The model under review builds one solid part; all positions refer to its coordinate system, in mm. Face numbers are marked on the shaded views. A direction names the side the tool comes from. Round coordinates to 2 decimals unless told otherwise and drop trailing zeros. Write each loop counter-clockwise with the first axis right and the second up, starting at its lowest first coordinate (ties: lowest second). Pieces come first, ordered by that corner, then holes. Notation, with made-up numbers: M 79.5,73.5 L 111.5,73.5 A27 cw 111.5,94.5 Z; hole C 20,-12.5 d8. An arc over 180 degrees is marked long. Write item = value, one per line. Start each with the question number.
Item 1: Take a section at B-B, the plane x = 0. Give the boundary of the cut face in (y, z), plus the area to 3 significant figures.
Item 2: Take a section at A-A, the plane y = 0. Give the boundary of the cut face in (x, z).
Item 3: For pin 1 Ø1.5 at (y, z) = (1, 18.5) entering from +X; pin 2 Ø1.5 at (x, y) = (0.5, 6.5) entering from +Z; pin 3 Ø9.5 at (x, y) = (0, 0) entering from -Z; pin 4 Ø1 at (x, z) = (-25, 17) entering from +Y, all flat-tipped, find the tip position at first contact; note any pin that passes through.
Item 4: Tool access review of the marked faces 4, 5 and 6: name each direction out of +Z, -Z, +X, -X, +Y, -Y from which nothing blocks a thin tool from reaching the whole face with its end or side.
Item 5: The part is to be moulded in two halves that separate along X. For the marked faces 1, 2 and 3, say which applies: +X half, -X half, draft (parallel to the pull), parting line (faces both ways), or undercut.
Item 6: To check wall thickness, follow line 1 along Y through (x, z) = (0, -0.7); line 2 along Z through (x, y) = (8, -5.75); line 3 along Y through (x, z) = (0, 2.3). State the ranges of each line that lie inside material, in increasing order.
Item 7: Take a section at C-C, the plane z = 0.75. Give the boundary of the cut face in (x, y), plus the area to 3 significant figures.
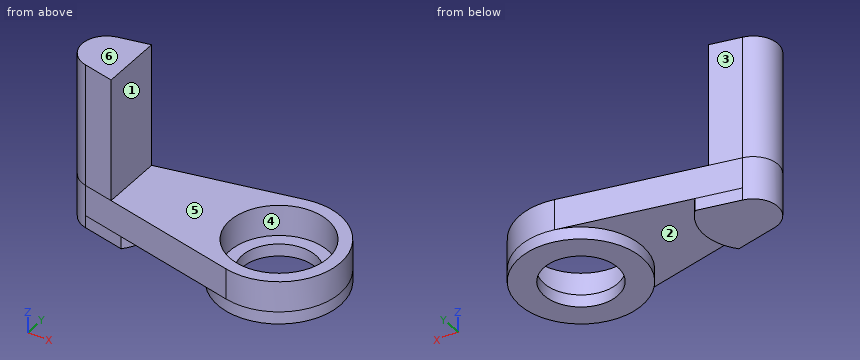
from build123d import *

# Parameters (mm, degrees)
SKETCH_R      = 8
PAD_DEPTH     = 5
PAD001_DEPTH  = 20
SKETCH002_R   = 10
SKETCH002_R_2 = 6
PAD002_DEPTH  = 2
PAD003_DEPTH  = 2


with BuildPart() as part:
    # Sketch → Pad (new body)
    with BuildSketch(Plane.XY):
        with BuildLine():
            ThreePointArc((-2.142857, -9.76771), (10, 0), (-2.142857, 9.76771))
            Line((-28.857143, 3.907084), (-2.142857, 9.76771))
            ThreePointArc((-28.857143, 3.907084), (-32, 0), (-28.857143, -3.907084))
            Line((-2.142857, -9.76771), (-28.857143, -3.907084))
        make_face()
        Circle(SKETCH_R, mode=Mode.SUBTRACT)
    extrude(amount=PAD_DEPTH)

    # Sketch001 (on Face7 of Pad) → Pad001 (join)
    with BuildSketch(Plane.XY.offset(5)):
        with BuildLine():
            ThreePointArc((-28.857143, 3.907084), (-32, -1.3e-05), (-28.857117, -3.90709))
            Line((-24, -4.972619), (-28.857117, -3.90709))
            Line((-24, -4.972619), (-24, 4.972653))
            Line((-24, 4.972653), (-28.857143, 3.907084))
        make_face()
    extrude(amount=PAD001_DEPTH)

    # Sketch002 → Pad002 (join)
    with BuildSketch(Plane(origin=(0, 0, 0), x_dir=(1, 0, 0), z_dir=(0, 0, -1))):
        Circle(SKETCH002_R)
        Circle(SKETCH002_R_2, mode=Mode.SUBTRACT)
    extrude(amount=PAD002_DEPTH)

    # Sketch003 (on Face7 of Pad002) → Pad003 (join)
    with BuildSketch(Plane(origin=(0, 0, 0), x_dir=(1, 0, 0), z_dir=(0, 0, -1))):
        with BuildLine():
            ThreePointArc((-28.857143, 3.907084), (-32, 0), (-28.857143, -3.907084))
            Line((-28.857143, -3.907084), (-22.089875, -5.391699))
            ThreePointArc((-22.089875, -5.391699), (-20, 0), (-22.089875, 5.391699))
            Line((-22.089875, 5.391699), (-28.857143, 3.907084))
        make_face()
    extrude(amount=PAD003_DEPTH)


solid = part.part
Response values:
q1.outline = M -10,-2 L -6,-2 L -6,0 L -8,0 L -8,5 L -10,5 Z; M 6,-2 L 10,-2 L 10,5 L 8,5 L 8,0 L 6,0 Z
q1.area = 36.0 mm2
q2.outline = M -32,-2 L -20,-2 L -20,0 L -10,0 L -10,-2 L -6,-2 L -6,0 L -8,0 L -8,5 L -24,5 L -24,25 L -32,25 Z; M 6,-2 L 10,-2 L 10,5 L 8,5 L 8,0 L 6,0 Z
q3.pin_1 = -24
q3.pin_2 = 0
q3.pin_3 = through
q3.pin_4 = 4.86
q4.face_4 = +Z
q4.face_5 = +Z, +X, +Y, -Y
q4.face_6 = +Z, +X, -X, +Y, -Y
q5.face_1 = +X half
q5.face_2 = undercut
q5.face_3 = -X half
q6.line_1 = -10 to -6, 6 to 10
q6.line_2 = -2 to 5
q6.line_3 = -10 to -8, 8 to 10
q7.outline = M -28.86,-3.91 L -2.14,-9.77 A10 ccw long -2.14,9.77 L -28.86,3.91 A4 ccw Z; hole C 0,0 d16
q7.area = 382 mm2
